Can you work these out from the model? Positions are in its coordinate system, mm. Face numbers are marked on the shaded views. A direction names the side the tool comes from. Round coordinates to 2 decimals unless told otherwise and drop trailing zeros. Order: outer loops, then holes, each group sorted by start corner. A loop starts at its lowest first (then second) coordinate and runs counter-clockwise, first axis right, second up.
Q1. Will these pins go through, and if not, where does the flat tip stop? P1, Ø4, axis at y = -26.5, z = 21, coming from the +X side; P2, Ø3, axis at x = 15.5, y = -15.5, coming from the +Z side; P3, Ø5, axis at x = 15.5, z = 4.5, coming from the +Y side; P4, Ø0.9, axis at x = -22.5, z = 7.5, coming from the +Y side.
Q2. If we section it at B-B (z = 8): Please give me the cut outline in (x, y), plus the area to 3 significant figures.
Q3. If we section it at A-A (y = 0): Please give me the cut outline in (x, z), plus the area to 4 significant figures.
Q4. For the marked faces 1, 2 and 3, which set-ups out of +Z, -Z, +X, -X, +Y, -Y let a thin tool reach every point of the face, with its end or its side?
Q5. If we section it at C-C (x = -15.5): Please give me the cut outline in (y, z), plus the area to 4 significant figures.
Q6. We'd pull the mould along X, two halves only. Please class the marked faces 4, 5, 6 and 7: pulls with the +X half, pulls with the -X half, needs draft (parallel to the pull), parting line crosses it, or undercut.
Q7. If we section it at D-D (y = -31.5): Please give me the cut outline in (x, z).
Q8. If I drill on line 1 (Y direction, x = 0, z = 4); line 2 (Y direction, x = -15, z = 3); line 3 (Z direction, x = -14.5, y = 6), over which ranges is the centre line in solid material (lowest first)?
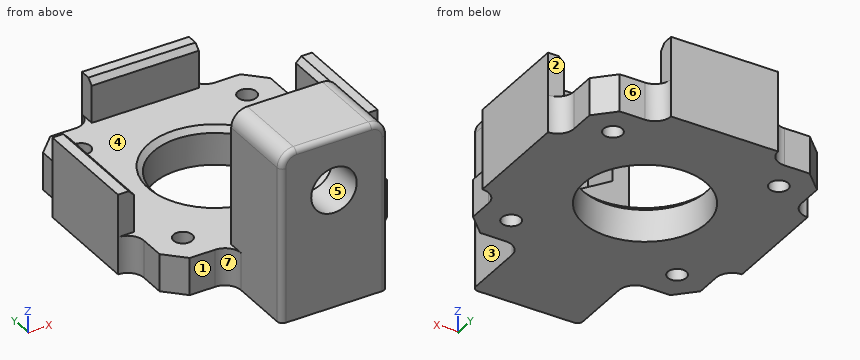
from build123d import *

# Parameters (mm, degrees)
ESQUISSE1_R             = 11.5
ESQUISSE1_R_2           = 1.75
BOSS_EXTRU_1_DEPTH      = 7
ESQUISSE2_W             = 20
ESQUISSE2_H             = 3
ESQUISSE2_W_2           = 3
ESQUISSE2_H_2           = 20
BOSS_EXTRU_2_DEPTH      = 15
ESQUISSE3_W             = 20
ESQUISSE3_H             = 15
BOSS_EXTRU_3_DEPTH      = 32
CONG_1_R                = 3
CONG_2_R                = 3
CHANFREIN1_SIZE         = 1
ESQUISSE4_R             = 4.25
ENL_V_MAT_EXTRU_1_DEPTH = 15
CONG_3_R                = 1
ENL_V_MAT_EXTRU_2_DEPTH = 7.5


with BuildPart() as part:
    # Esquisse1 → Boss.-Extru.1 (new body)
    with BuildSketch(Plane.XY):
        Polygon((-17.749999999, 21.249999999), (-21.249999999, 17.749999999), (-21.249999999, -17.749999999), (-17.749999999, -21.250000001), (17.749999999, -21.250000001), (21.249999999, -17.749999999), (21.249999999, 17.749999999), (17.749999999, 21.249999999), align=None)
        Circle(ESQUISSE1_R, mode=Mode.SUBTRACT)
        with Locations((-15.5, 15.5)):
            Circle(ESQUISSE1_R_2, mode=Mode.SUBTRACT)
        with Locations((15.5, 15.5)):
            Circle(ESQUISSE1_R_2, mode=Mode.SUBTRACT)
        with Locations((15.5, -15.5)):
            Circle(ESQUISSE1_R_2, mode=Mode.SUBTRACT)
        with Locations((-15.5, -15.5)):
            Circle(ESQUISSE1_R_2, mode=Mode.SUBTRACT)
    extrude(amount=BOSS_EXTRU_1_DEPTH)

    # Esquisse2 → Boss.-Extru.2 (add)
    with BuildSketch(Plane(origin=(0, 0, 0), x_dir=(-1, 0, 0), z_dir=(0, 0, -1))):
        with Locations((0, 22.749999999)):
            Rectangle(ESQUISSE2_W, ESQUISSE2_H)
        with Locations((22.749999999, 0)):
            Rectangle(ESQUISSE2_W_2, ESQUISSE2_H_2)
        with Locations((-22.749999999, 0)):
            Rectangle(ESQUISSE2_W_2, ESQUISSE2_H_2)
    extrude(amount=-BOSS_EXTRU_2_DEPTH)

    # Esquisse3 → Boss.-Extru.3 (add)
    with BuildSketch(Plane(origin=(0, 0, 0), x_dir=(-1, 0, 0), z_dir=(0, 0, -1))):
        with Locations((0, -28.750000001)):
            Rectangle(ESQUISSE3_W, ESQUISSE3_H)
    extrude(amount=-BOSS_EXTRU_3_DEPTH)

    # Congé1
    cong_1_edges = [part.edges().sort_by_distance(p)[0] for p in [
        (-21.249999999, -10, 3.5),
        (-21.249999999, 10, 3.5),
        (-10, 21.249999999, 3.5),
        (10, 21.249999999, 3.5),
        (21.249999999, 10, 3.5),
        (21.249999999, -10, 3.5),
        (10, -21.250000001, 3.5),
        (-10, -21.250000001, 3.5),
    ]]
    fillet(cong_1_edges, radius=CONG_1_R - 0.0001)  # a hair under: the kernel refuses the full size

    # Congé2
    cong_2_edges = [part.edges().sort_by_distance(p)[0] for p in [
        (10, -28.750000001, 32),
        (-10, -28.750000001, 32),
    ]]
    fillet(cong_2_edges, radius=CONG_2_R)

    # Chanfrein1
    chanfrein1_edges = [part.edges().sort_by_distance(p)[0] for p in [
        (-11.5, 0, 7),
        (0, 21.249999999, 15),
        (-21.249999999, 0, 15),
        (21.249999999, 0, 15),
    ]]
    chamfer(chanfrein1_edges, length=CHANFREIN1_SIZE)

    # Esquisse4 → Enlèv. mat.-Extru.1 (cut)
    with BuildSketch(Plane(origin=(0, -36.250000001, 0), x_dir=(-1, 0, 0), z_dir=(0, -1, 0))):
        with Locations(Location((0, -22, 0), (0, 0, 90))):
            Circle(ESQUISSE4_R)
    extrude(amount=-ENL_V_MAT_EXTRU_1_DEPTH, mode=Mode.SUBTRACT)

    # Congé3
    cong_3_edges = [part.edges().sort_by_distance(p)[0] for p in [
        (10, -36.250000001, 14.5),
        (0, -36.250000001, 32),
        (-10, -36.250000001, 14.5),
        (-9.121320344, -36.250000001, 31.121320344),
        (9.121320344, -36.250000001, 31.121320344),
    ]]
    fillet(cong_3_edges, radius=CONG_3_R)

    # Esquisse5 → Enlèv. mat.-Extru.2 (cut)
    with BuildSketch(Plane(origin=(0, -21.250000001, 0), x_dir=(1, 0, 0), z_dir=(0, 1, 0))):
        Polygon((0, -30.082903769), (7, -26.041451884), (7, -17.958548116), (0, -13.917096231), (-7, -17.958548116), (-7, -26.041451884), align=None)
    extrude(amount=-ENL_V_MAT_EXTRU_2_DEPTH, mode=Mode.SUBTRACT)


solid = part.part
Solution:
1. P1: stops at x = 10
1. P2: passes through
1. P3: stops at y = 21.25
1. P4: stops at y = 10
2. outline: (-24.25, -10) - (-21.25, -10) - (-21.25, 10) - (-24.25, 10) - close; (-10, -35.25) arc R1 ccw to (-9, -36.25) - (9, -36.25) arc R1 ccw to (10, -35.25) - (10, -21.25) - (-10, -21.25) - close; (-10, 21.25) - (10, 21.25) - (10, 24.25) - (-10, 24.25) - close; (21.25, -10) - (24.25, -10) - (24.25, 10) - (21.25, 10) - close
2. area: 480 mm2
3. outline: (-24.25, 0) - (-11.5, 0) - (-11.5, 6) - (-12.5, 7) - (-21.25, 7) - (-21.25, 14) - (-22.25, 15) - (-24.25, 15) - close; (11.5, 0) - (24.25, 0) - (24.25, 15) - (22.25, 15) - (21.25, 14) - (21.25, 7) - (12.5, 7) - (11.5, 6) - close
3. area: 224.5 mm2
4. face 1: +Z, -Z, -X, -Y
4. face 2: +Z, +X, -X, +Y
4. face 3: +Z, +X, -Y
5. outline: (-21.25, 0) - (-17.25, 0) - (-17.25, 7) - (-21.25, 7) - close; (-13.75, 0) - (13.75, 0) - (13.75, 7) - (-13.75, 7) - close; (17.25, 0) - (21.25, 0) - (21.25, 7) - (17.25, 7) - close
5. area: 248.5 mm2
6. face 4: undercut
6. face 5: undercut
6. face 6: needs draft
6. face 7: pulls with the -X half
7. outline: (-10, 0) - (10, 0) - (10, 29) arc R3 ccw to (7, 32) - (-7, 32) arc R3 ccw to (-10, 29) - close; hole circle Ø8.5 at (0, 22)
8. line 1: y = -36.25 to -11.5, 11.5 to 24.25
8. line 2: y = -21.25 to -17.18, -13.82 to 13.82, 17.18 to 21.25
8. line 3: z = 0 to 7
